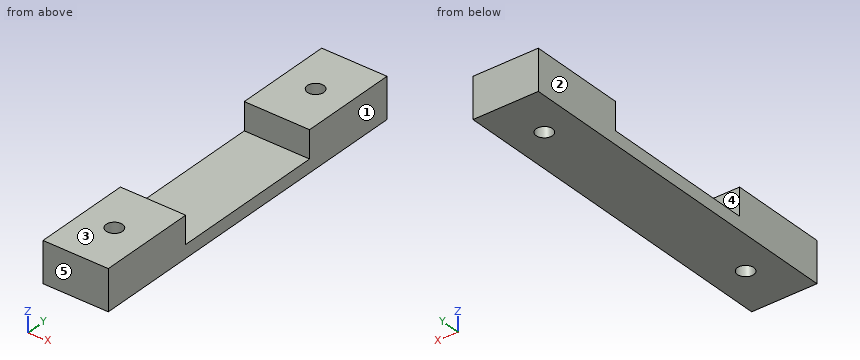
```python
from build123d import *

# Parameters (mm, degrees)
SKETCH_1_W          = 10
SKETCH_1_H          = 54
EXTRUDE_1_DEPTH     = 2
SKETCH_2_W          = 10
SKETCH_2_H          = 15
EXTRUDE_2_DEPTH     = 4.2
SKETCH_3_R          = 1.25
CUT_EXTRUDE_1_DEPTH = 83.01490969


with BuildPart() as part:
    # 草圖1 → 填料-伸長1 (new body)
    with BuildSketch(Plane.XY):
        with Locations((-56.635565313, 26.75)):
            Rectangle(SKETCH_1_W, SKETCH_1_H)
    extrude(amount=EXTRUDE_1_DEPTH)

    # 草圖2 → 填料-伸長2 (add)
    with BuildSketch(Plane.XY.offset(2)):
        with Locations((-56.635565313, 7.25)):
            Rectangle(SKETCH_2_W, SKETCH_2_H)
        with Locations((-56.635565313, 46.25)):
            Rectangle(SKETCH_2_W, SKETCH_2_H)
    extrude(amount=EXTRUDE_2_DEPTH)

    # 草圖3 → 除料-伸長1 (cut, through all)
    with BuildSketch(Plane.XY.offset(6.2)):
        with Locations((-56.635565313, 7.25)):
            Circle(SKETCH_3_R)
        with Locations((-56.635565313, 46.25)):
            Circle(SKETCH_3_R)
    extrude(amount=-CUT_EXTRUDE_1_DEPTH, mode=Mode.SUBTRACT)


solid = part.part
```
Here's how the part is built. I have some questions about the finished solid (model axes, mm). Face numbers are marked on the shaded views. A direction names the side the tool comes from. Round coordinates to 2 decimals unless told otherwise and drop trailing zeros. Order: outer loops, then holes, each group sorted by start corner. A loop starts at its lowest first (then second) coordinate and runs counter-clockwise, first axis right, second up. Notation, with made-up numbers: (2.25, 46) -> (23.25, 46) arc R13 cw to (23.25, 58) -> close; hole circle Ø4 at (-8.5, 8.5). An arc over 180 degrees is marked (long way). Use a Markdown table: item, result. Add a question column.
(1) For the marked faces 4 and 5, which set-ups out of +Z, -Z, +X, -X, +Y, -Y let a thin tool reach every point of the face, with its end or its side?
(2) Suppose I cut it at D-D, the plane x = -61. Please give me the cut outline in (y, z), and give its area (3 significant figures).
(3) I need wall thicknesses on line 1 along Y through (x, z) = (-56.5, 5.75); line 2 along Y through (x, z) = (-56.75, 0.5); line 3 along Y through (x, z) = (-58, 5.75). Which ranges of each line are inside material? Lowest first, please.
(4) Suppose I cut it at B-B, the plane y = 7.25. Please give me the cut outline in (x, z).
(5) Suppose I cut it at C-C, the plane x = -56. Please give me the cut outline in (y, z), and give its area (3 significant figures).
(6) If we mould it in two halves opening along X, with no side actions, what happens to the marked faces 1, 2 and 3? For each: released by +X, released by -X, zero draft, split by the parting line, or undercut.
(7) Suppose I cut it at A-A, the plane z = 4.25. Please give me the cut outline in (x, y), and give its area (3 significant figures).
(8) For pin 1 Ø3 at (x, y) = (-56.64, 46.25) entering from -Z; pin 2 Ø3 at (x, y) = (-55, 23) entering from +Z, each with a flat end and sliding along its axis, tell me the tip position at first contact or that it passes through.
Verdict:
| question | item | result |
|---|---|---|
| 1 | face 4 | +Z, +X, -X |
| 1 | face 5 | +Z, -Z, +X, -X, -Y |
| 2 | outline | (-0.25, 0) -> (53.75, 0) -> (53.75, 6.2) -> (38.75, 6.2) -> (38.75, 2) -> (14.75, 2) -> (14.75, 6.2) -> (-0.25, 6.2) -> close |
| 2 | area | 234 mm2 |
| 3 | line 1 | -0.25 to 6.01, 8.49 to 14.75, 38.75 to 45.01, 47.49 to 53.75 |
| 3 | line 2 | -0.25 to 6.01, 8.49 to 45.01, 47.49 to 53.75 |
| 3 | line 3 | -0.25 to 14.75, 38.75 to 53.75 |
| 4 | outline | (-61.64, 0) -> (-57.89, 0) -> (-57.89, 6.2) -> (-61.64, 6.2) -> close; (-55.39, 0) -> (-51.64, 0) -> (-51.64, 6.2) -> (-55.39, 6.2) -> close |
| 5 | outline | (-0.25, 0) -> (6.17, 0) -> (6.17, 6.2) -> (-0.25, 6.2) -> close; (8.33, 0) -> (45.17, 0) -> (45.17, 6.2) -> (38.75, 6.2) -> (38.75, 2) -> (14.75, 2) -> (14.75, 6.2) -> (8.33, 6.2) -> close; (47.33, 0) -> (53.75, 0) -> (53.75, 6.2) -> (47.33, 6.2) -> close |
| 5 | area | 207 mm2 |
| 6 | face 1 | released by +X |
| 6 | face 2 | released by -X |
| 6 | face 3 | zero draft |
| 7 | outline | (-61.64, -0.25) -> (-51.64, -0.25) -> (-51.64, 14.75) -> (-61.64, 14.75) -> close; (-61.64, 38.75) -> (-51.64, 38.75) -> (-51.64, 53.75) -> (-61.64, 53.75) -> close; hole circle Ø2.5 at (-56.64, 7.25); hole circle Ø2.5 at (-56.64, 46.25) |
| 7 | area | 290 mm2 |
| 8 | pin 1 | z = 0 |
| 8 | pin 2 | z = 2 |
